Geometry check sheet. Reference: the model listing, model coordinates, mm. Face numbers are marked on the shaded views. A direction names the side the tool comes from. Give positions to 0.01 mm unless a question says otherwise; leave off trailing zeros. Loops run counter-clockwise (first coordinate to the right, second up) from the corner with the lowest first, then second, coordinate; pieces in that order, holes last. Notation, with made-up numbers: (13.25, 24.25) -> (67.25, 24.25) arc R22 cw to (67.25, 40.25) -> close; hole circle Ø6 at (14, 18). An arc over 180 degrees is marked (long way). One line per item, written item: value. Start each with the question number.
(1) Scan lines: line 1 along Y through (x, z) = (-15.5, 7); line 2 along Y through (x, z) = (-15.5, 7.5); line 3 along X through (y, z) = (-15, 5). Record each from-to range of solid material in increasing order. Write a range as from..to.
(2) Sectioned sample at B-B, the plane z = 34.5. Record the cut outline in (x, y).
(3) Tool access check on the marked faces 1, 2, 3 and 4. Record the directions out of +Z, -Z, +X, -X, +Y, -Y that give a thin tool (end or side, any length) a straight path to the whole face; none if there is none.
(4) Sectioned sample at D-D, the plane y = 0. Record the cut outline in (x, z).
(5) Gauge pin test, flat ends, axial feed: pin 1 Ø2 at (x, y) = (14, -7) entering from -Z; pin 2 Ø17.5 at (x, z) = (7, 14) entering from -Y; pin 3 Ø1.5 at (y, z) = (-24, 34.5) entering from -X. Record the tip position at first contact, or that the pin passes through.
(6) Sectioned sample at C-C, the plane x = 0. Record the cut outline in (y, z).
(7) Draft check along Z on the marked faces 5, 6 and 7. Enter one of: pulls with the +Z half, pulls with the -Z half, needs draft (parallel to the pull), parting line crosses it, or undercut.
(8) Sectioned sample at A-A, the plane z = 3. Record the cut outline in (x, y).
from build123d import *

# Parameters (mm, degrees)
RESSALTO_EXTRUS_O1_DEPTH   = 38
CORTE_EXTRUS_O_FINA1_START = -30.8
CORTE_EXTRUS_O_FINA1_DEPTH = 21.6
ESBO_O3_R                  = 2.25
RESSALTO_EXTRUS_O2_DEPTH   = 20
ESBO_O4_R                  = 10
RESSALTO_EXTRUS_O3_DEPTH   = 2
ESBO_O5_R                  = 1.5
CORTE_EXTRUS_O1_DEPTH      = 10
ESBO_O7_W                  = 16
ESBO_O7_H                  = 5
RESSALTO_EXTRUS_O4_DEPTH   = 10


# Read off the part's stored shape, not the designer's step: Corte-Extrusão-Fina1
with BuildPart() as part:
    # Esboço1 → Ressalto-extrusão1 (new body)
    with BuildSketch(Plane.XY):
        Polygon((-21, -15.592171873), (-15.984175996, -21), (15.592171873, -21), (21, -15.984175996), (21, 15.592171873), (15.984175996, 21), (-15.592171873, 21), (-21, 15.984175996), align=None)
    extrude(amount=RESSALTO_EXTRUS_O1_DEPTH)

    # Corte-Extrusão-Fina1 outline → Corte-Extrusão-Fina1 (cut)
    with BuildSketch(Plane.XY.offset(38).offset(CORTE_EXTRUS_O_FINA1_START)):
        Polygon((15.592171873, -21), (21, -15.984175996), (21, 15.592171873), (15.984175996, 21), (-15.592171873, 21), (-21, 15.984175996), (-21, -15.592171873), (-15.984175996, -21), align=None)
        Polygon((14.605339059, 20.75), (20.75, 14.605339059), (20.75, -14.605339059), (14.605339059, -20.75), (-14.605339059, -20.75), (-20.75, -14.605339059), (-20.75, 14.605339059), (-14.605339059, 20.75), align=None, mode=Mode.SUBTRACT)
    extrude(amount=CORTE_EXTRUS_O_FINA1_DEPTH, mode=Mode.SUBTRACT)

    # Esboço3 → Ressalto-extrusão2 (add)
    with BuildSketch(Plane(origin=(0, 0, 0), x_dir=(-1, 0, 0), z_dir=(0, 0, -1))):
        with Locations(Location((0, 0, 0), (0, 0, 180))):
            Circle(ESBO_O3_R)
    extrude(amount=RESSALTO_EXTRUS_O2_DEPTH)

    # Esboço4 → Ressalto-extrusão3 (add)
    with BuildSketch(Plane(origin=(0, 0, 0), x_dir=(-1, 0, 0), z_dir=(0, 0, -1))):
        with Locations(Location((0, 0, 0), (0, 0, 180))):
            Circle(ESBO_O4_R)
    extrude(amount=RESSALTO_EXTRUS_O3_DEPTH)

    # Esboço5 → Corte-extrusão1 (cut)
    with BuildSketch(Plane(origin=(0, 0, 0), x_dir=(-1, 0, 0), z_dir=(0, 0, -1))):
        with Locations((15.5, -15.5)):
            Circle(ESBO_O5_R)
        with Locations((-15.5, -15.5)):
            Circle(ESBO_O5_R)
        with Locations((-15.5, 15.5)):
            Circle(ESBO_O5_R)
        with Locations((15.5, 15.5)):
            Circle(ESBO_O5_R)
    extrude(amount=-CORTE_EXTRUS_O1_DEPTH, mode=Mode.SUBTRACT)

    # Esboço7 → Ressalto-extrusão4 (add)
    with BuildSketch(Plane.XZ.offset(21)):
        with Locations((-0.196002062, 35.5)):
            Rectangle(ESBO_O7_W, ESBO_O7_H)
    extrude(amount=RESSALTO_EXTRUS_O4_DEPTH)


solid = part.part
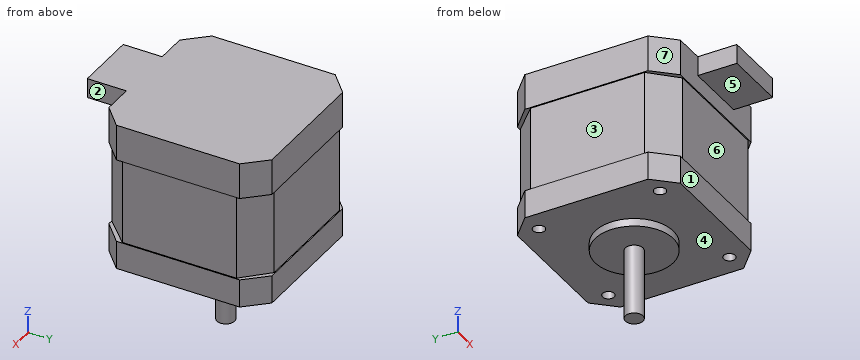
Calculated:
1. line 1: y = -21..-17, -14..14, 17..21
1. line 2: y = -19.86..-17, -14..14, 17..19.86
1. line 3: x = -21..-16.91, -14.09..14.09, 16.91..21
2. outline: (-21, -15.59) -> (-15.98, -21) -> (-8.2, -21) -> (-8.2, -31) -> (7.8, -31) -> (7.8, -21) -> (15.59, -21) -> (21, -15.98) -> (21, 15.59) -> (15.98, 21) -> (-15.59, 21) -> (-21, 15.98) -> close
3. face 1: -Z, +X, -X, -Y
3. face 2: +Z, -Z, +X, -Y
3. face 3: -X, +Y, -Y
3. face 4: -Z
4. outline: (-21, 0) -> (-10, 0) -> (-10, -2) -> (-2.25, -2) -> (-2.25, -20) -> (2.25, -20) -> (2.25, -2) -> (10, -2) -> (10, 0) -> (21, 0) -> (21, 7.2) -> (20.75, 7.2) -> (20.75, 28.8) -> (21, 28.8) -> (21, 38) -> (-21, 38) -> (-21, 28.8) -> (-20.75, 28.8) -> (-20.75, 7.2) -> (-21, 7.2) -> close
5. pin 1: stops at z = 0
5. pin 2: stops at y = -21
5. pin 3: stops at x = -8.2
6. outline: (-31, 33) -> (-21, 33) -> (-21, 28.8) -> (-20.75, 28.8) -> (-20.75, 7.2) -> (-21, 7.2) -> (-21, 0) -> (-10, 0) -> (-10, -2) -> (-2.25, -2) -> (-2.25, -20) -> (2.25, -20) -> (2.25, -2) -> (10, -2) -> (10, 0) -> (21, 0) -> (21, 7.2) -> (20.75, 7.2) -> (20.75, 28.8) -> (21, 28.8) -> (21, 38) -> (-31, 38) -> close
7. face 5: pulls with the -Z half
7. face 6: undercut
7. face 7: needs draft
8. outline: (-21, -15.59) -> (-15.98, -21) -> (15.59, -21) -> (21, -15.98) -> (21, 15.59) -> (15.98, 21) -> (-15.59, 21) -> (-21, 15.98) -> close; hole circle Ø3 at (-15.5, -15.5); hole circle Ø3 at (-15.5, 15.5); hole circle Ø3 at (15.5, -15.5); hole circle Ø3 at (15.5, 15.5)
